Here's how the part is built. I have some questions about the finished solid (model axes, mm). A direction names the side the tool comes from. Coordinates: 2 decimals unless noted, no trailing zeros. Write each loop counter-clockwise with the first axis right and the second up, starting at its lowest first coordinate (ties: lowest second). Pieces come first, ordered by that corner, then holes. Notation, with made-up numbers: (-21, 75.25) -> (16, 75.25) arc R24 cw to (16, 107.25) -> close; hole circle Ø1 at (-22.5, 31). An arc over 180 degrees is marked (long way). Use a Markdown table: item, result. Add a question column.
Item 1: If I drill on line 1 along X through (y, z) = (375.25, -80); line 2 along Y through (x, z) = (-1065, -6); line 3 along Z through (x, y) = (-1040, 566) (3 decimals), over which ranges is the centre line in solid material (lowest first)? Write a range as from..to.
Item 2: On a 3-axis mill with a long thin cutter (end or side, diameter ignored), from which of +Z, -Z, +X, -X, +Y, -Y can I reach the whole of each face in a straight line? I mean faces 1 (the flat face through (-990, 513.97, -1)), 2 (the flat face through (-990, 620, -2)), 3 (the flat face through (-909.138, 456, 2)). Say none if no direction works.
Item 3: Imagine slicing it at B-B, the plane z = 0. Write out the boundary of the cut face in (x, y).
Item 4: Will these pins go through, and if not, where does the flat tip stop? pin 1 Ø1.5 at (y, z) = (405, 76) entering from -X; pin 2 Ø3 at (y, z) = (441.5, 46) entering from +X.
Item 5: Imagine slicing it at D-D, the plane y = 409. Write out the boundary of the cut face in (x, z), and give its area (3 significant figures).
Item 6: If we mould it in two halves opening along X, with no side actions, what happens to faces 4 (the cylindrical face through (-1001.93, 487.74, -58.71)), 5 (the conical face through (-964.263, 624.757, 51.444)), 6 (the flat face through (-853.583, 380, -2))? For each: pulls with the +X half, pulls with the -X half, needs draft (parallel to the pull), parting line crosses it, or undercut.
Item 7: Imagine slicing it at C-C, the plane y = 535. Write out the boundary of the cut face in (x, z) (3 decimals).
Item 8: Imagine slicing it at A-A, the plane x = -929.5. Write out the boundary of the cut face in (y, z) (3 decimals).
```python
from build123d import *

# Parameters (mm, degrees)
SKETCH_1_W                    = 221.417168307
SKETCH_1_H                    = 240
EXTRUDE_1_DEPTH               = 20
SKETCH_2_W                    = 160.152997215
SKETCH_2_H                    = 240
EXTRUDE_2_DEPTH               = 230
SKETCH_3_W                    = 214.21
SKETCH_3_H                    = 95.18
CUT_EXTRUDE_1_DEPTH           = 660.673983169
HOLE_WIZARD_M30_1_D           = 26.5
HOLE_WIZARD_M30_1_DEPTH       = 50
HOLE_WIZARD_M30_1_CSINK_D     = 30.05
HOLE_WIZARD_M30_1_CSINK_ANGLE = 90
HOLE_WIZARD_M30_1_TIP         = 7.961403202
SKETCH_11_R                   = 15.562071092
CUT_EXTRUDE_3_DEPTH           = 20
SKETCH_12_R                   = 25
EXTRUDE_3_DEPTH               = 10
SKETCH_13_R                   = 15.562071092
CUT_EXTRUDE_4_DEPTH           = 29.5
SKETCH_14_W                   = 25
SKETCH_14_H                   = 240
EXTRUDE_4_DEPTH               = 20
SKETCH_15_R                   = 10
CUT_EXTRUDE_5_DEPTH           = 25
CHAMFER_1_SIZE                = 5
FILLET_1_R                    = 10
FILLET_2_R                    = 5


with BuildPart() as part:
    # 草图1 → 凸台-拉伸1 (new body)
    with BuildSketch(Plane(origin=(0, 370, 0), x_dir=(1, 0, 0), z_dir=(0, 1, 0))):
        with Locations((-989.291415847, 0)):
            Rectangle(SKETCH_1_W, SKETCH_1_H)
    extrude(amount=EXTRUDE_1_DEPTH)

    # 草图2 → 凸台-拉伸2 (add)
    with BuildSketch(Plane(origin=(0, 390, 0), x_dir=(1, 0, 0), z_dir=(0, 1, 0))):
        with Locations((-989.214917238, 0)):
            Rectangle(SKETCH_2_W, SKETCH_2_H)
    extrude(amount=EXTRUDE_2_DEPTH)

    # 草图3 → 切除-拉伸1 (cut, through all)
    with BuildSketch(Plane.ZY.offset(1069.291415846)):
        with Locations((0, 561.56)):
            Rectangle(SKETCH_3_W, SKETCH_3_H)
    extrude(amount=-CUT_EXTRUDE_1_DEPTH, mode=Mode.SUBTRACT)

    # M30 螺纹孔1
    with Locations(Plane(origin=(0, 513.97, 0), x_dir=(1, 0, 0), z_dir=(0, 1, 0))):
        with Locations((-989.291415846, 54.73), (-989.291415846, -54.73)):
            CounterSinkHole(HOLE_WIZARD_M30_1_D / 2, HOLE_WIZARD_M30_1_CSINK_D / 2, depth=HOLE_WIZARD_M30_1_DEPTH, counter_sink_angle=HOLE_WIZARD_M30_1_CSINK_ANGLE)
            with Locations((0, 0, -(HOLE_WIZARD_M30_1_DEPTH + HOLE_WIZARD_M30_1_TIP / 2))):  # 118° drill point
                Cone(0, HOLE_WIZARD_M30_1_D / 2, HOLE_WIZARD_M30_1_TIP, mode=Mode.SUBTRACT)

    # 草图11 → 切除-拉伸3 (cut)
    with BuildSketch(Plane(origin=(0, 620, 0), x_dir=(1, 0, 0), z_dir=(0, 1, 0))):
        with Locations(Location((-989.291415846, 54.73, 0), (0, 0, 270))):
            Circle(SKETCH_11_R)
        with Locations(Location((-989.291415846, -54.73, 0), (0, 0, 270))):
            Circle(SKETCH_11_R)
    extrude(amount=-CUT_EXTRUDE_3_DEPTH, mode=Mode.SUBTRACT)

    # 草图12 → 凸台-拉伸3 (add)
    with BuildSketch(Plane(origin=(0, 620, 0), x_dir=(1, 0, 0), z_dir=(0, 1, 0))):
        with Locations(Location((-989.291415846, 54.73, 0), (0, 0, 270))):
            Circle(SKETCH_12_R)
        with Locations(Location((-989.291415846, -54.73, 0), (0, 0, 270))):
            Circle(SKETCH_12_R)
    extrude(amount=EXTRUDE_3_DEPTH)

    # 草图13 → 切除-拉伸4 (cut, symmetric)
    with BuildSketch(Plane(origin=(0, 630, 0), x_dir=(1, 0, 0), z_dir=(0, 1, 0))):
        with Locations(Location((-989.291415846, 54.73, 0), (0, 0, 270))):
            Circle(SKETCH_13_R)
        with Locations(Location((-989.291415846, -54.73, 0), (0, 0, 270))):
            Circle(SKETCH_13_R)
    extrude(amount=CUT_EXTRUDE_4_DEPTH, both=True, mode=Mode.SUBTRACT)

    # 草图14 → 凸台-拉伸4 (add)
    with BuildSketch(Plane.XZ.offset(-370)):
        with Locations((-1112.5, 0)):
            Rectangle(SKETCH_14_W, SKETCH_14_H)
        with Locations((-866.082831693, 0)):
            Rectangle(SKETCH_14_W, SKETCH_14_H)
    extrude(amount=-EXTRUDE_4_DEPTH)

    # 草图15 → 切除-拉伸5 (cut, symmetric)
    with BuildSketch(Plane(origin=(0, 390, 0), x_dir=(1, 0, 0), z_dir=(0, 1, 0))):
        with Locations(Location((-1097.145707923, -80, 0), (0, 0, 270))):
            Circle(SKETCH_15_R)
        with Locations(Location((-1097.145707923, 80, 0), (0, 0, 270))):
            Circle(SKETCH_15_R)
    cut_extrude_5 = extrude(amount=CUT_EXTRUDE_5_DEPTH, both=True, mode=Mode.SUBTRACT)

    # 镜向1: 切除-拉伸5 across plane
    add(cut_extrude_5.mirror(Plane.ZY.offset(989.214917239)), mode=Mode.SUBTRACT)

    # 倒角1
    chamfer_1_edges = [part.edges().sort_by_distance(p)[0] for p in [
        (-1069.291415846, 390, 0),
        (-909.138418631, 390, 0),
        (-989.291415846, 620, -79.73),
        (-989.291415846, 620, 29.73),
    ]]
    chamfer(chamfer_1_edges, length=CHAMFER_1_SIZE)

    # 圆角1
    fillet_1_edges = [part.edges().sort_by_distance(p)[0] for p in [
        (-853.582831693, 380, -120),
        (-853.582831693, 380, 120),
        (-1125, 380, 120),
        (-1125, 380, -120),
    ]]
    fillet(fillet_1_edges, radius=FILLET_1_R)

    # 圆角2
    fillet_2_edges = [part.edges().sort_by_distance(p)[0] for p in [
        (-1069.291415846, 507.5, -120),
        (-1069.291415846, 507.5, 120),
        (-909.138418631, 507.5, 120),
        (-909.138418631, 507.5, -120),
    ]]
    fillet(fillet_2_edges, radius=FILLET_2_R)


solid = part.part
```
Ans:
| question | item | result |
|---|---|---|
| 1 | line 1 | x = -1125..-1107.15, -1087.15..-891.28, -871.28..-853.58 |
| 1 | line 2 | y = 370..513.97, 609.15..620 |
| 1 | line 3 | z = -120..-107.105, 107.105..120 |
| 2 | face 1 | +X, -X |
| 2 | face 2 | +Y |
| 2 | face 3 | +Z, -Z, +X, +Y |
| 3 | outline | (-1125, 370) -> (-853.58, 370) -> (-853.58, 390) -> (-904.14, 390) -> (-909.14, 395) -> (-909.14, 513.97) -> (-1069.29, 513.97) -> (-1069.29, 395) -> (-1074.29, 390) -> (-1125, 390) -> close; (-1069.29, 609.15) -> (-909.14, 609.15) -> (-909.14, 620) -> (-1069.29, 620) -> close |
| 4 | pin 1 | stops at x = -1069.29 |
| 4 | pin 2 | stops at x = -909.14 |
| 5 | outline | (-1069.29, -115) arc R5 ccw to (-1064.29, -120) -> (-914.14, -120) arc R5 ccw to (-909.14, -115) -> (-909.14, 115) arc R5 ccw to (-914.14, 120) -> (-1064.29, 120) arc R5 ccw to (-1069.29, 115) -> close |
| 5 | area | 38,400 mm^2 |
| 6 | face 4 | undercut |
| 6 | face 5 | parting line crosses it |
| 6 | face 6 | pulls with the +X half |
| 7 | outline | (-1069.291, -115) arc R5 ccw to (-1064.291, -120) -> (-914.138, -120) arc R5 ccw to (-909.138, -115) -> (-909.138, -107.105) -> (-1069.291, -107.105) -> close; (-1069.291, 107.105) -> (-909.138, 107.105) -> (-909.138, 115) arc R5 ccw to (-914.138, 120) -> (-1064.291, 120) arc R5 ccw to (-1069.291, 115) -> close |
| 8 | outline | (370, -120) -> (620, -120) -> (620, 120) -> (370, 120) -> close; hole (513.97, -107.105) -> (609.15, -107.105) -> (609.15, 107.105) -> (513.97, 107.105) -> close |
